```python
from build123d import *

# Parameters (mm, degrees)
SKETCH_4_W          = 88.9
SKETCH_4_H          = 88.9
SKETCH_4_R          = 1.5
SKETCH_4_W_2        = 38.1
SKETCH_4_H_2        = 3
SKETCH_4_W_3        = 3
SKETCH_4_H_3        = 38.1
EXTRUDE_1_DEPTH     = 3
SKETCH_6_W          = 88.9
SKETCH_6_H          = 3
EXTRUDE_2_DEPTH     = 24.13
SKETCH_7_W          = 3
SKETCH_7_H          = 7.62
CUT_EXTRUDE_1_DEPTH = 3


with BuildPart() as part:
    # 스케치4 → 보스-돌출1 (new body)
    with BuildSketch(Plane(origin=(0, 0, 0), x_dir=(1, 0, 0), z_dir=(0, 1, 0))):
        Rectangle(SKETCH_4_W, SKETCH_4_H)
        with Locations(Location((-41.275, 41.275, 0), (0, 0, 270))):
            Circle(SKETCH_4_R, mode=Mode.SUBTRACT)
        with Locations(Location((41.275, 41.275, 0), (0, 0, 270))):
            Circle(SKETCH_4_R, mode=Mode.SUBTRACT)
        with Locations(Location((41.275, -41.275, 0), (0, 0, 270))):
            Circle(SKETCH_4_R, mode=Mode.SUBTRACT)
        with Locations(Location((-41.275, -41.275, 0), (0, 0, 270))):
            Circle(SKETCH_4_R, mode=Mode.SUBTRACT)
        with Locations((0, 36.6)):
            Rectangle(SKETCH_4_W_2, SKETCH_4_H_2, mode=Mode.SUBTRACT)
        with Locations((36.6, 0)):
            Rectangle(SKETCH_4_W_3, SKETCH_4_H_3, mode=Mode.SUBTRACT)
        with Locations((0, -36.6)):
            Rectangle(SKETCH_4_W_2, SKETCH_4_H_2, mode=Mode.SUBTRACT)
        with Locations((-36.6, 0)):
            Rectangle(SKETCH_4_W_3, SKETCH_4_H_3, mode=Mode.SUBTRACT)
    extrude(amount=EXTRUDE_1_DEPTH)

    # 스케치6 → 보스-돌출2 (add)
    with BuildSketch(Plane(origin=(44.45, 0, 0), x_dir=(0, 0, -1), z_dir=(1, 0, 0))):
        with Locations((0, 1.5)):
            Rectangle(SKETCH_6_W, SKETCH_6_H)
    extrude(amount=EXTRUDE_2_DEPTH)

    # 스케치7 → 컷-돌출1 (cut)
    with BuildSketch(Plane(origin=(0, 3, 0), x_dir=(1, 0, 0), z_dir=(0, 1, 0))):
        with Locations((-13.1, -28.21025)):
            Rectangle(SKETCH_7_W, SKETCH_7_H)
    extrude(amount=-CUT_EXTRUDE_1_DEPTH, mode=Mode.SUBTRACT)


solid = part.part
```
Geometry check sheet. Reference: the model listing, model coordinates, mm. A direction names the side the tool comes from. Round coordinates to 2 decimals unless told otherwise and drop trailing zeros. Loops run counter-clockwise (first coordinate to the right, second up) from the corner with the lowest first, then second, coordinate; pieces in that order, holes last. Notation, with made-up numbers: (88.25, 49) - (143.25, 49) arc R23 ccw to (143.25, 75) - close; hole circle Ø6 at (11, -17). An arc over 180 degrees is marked (long way). Use a Markdown table: item, result.
Q1. Cross-section at C-C on y = 1.9. State how many separate pieces and enclosed holes the cut face has, plus the area to 3 significant figures.
Solutions:
| item | result |
|---|---|
| separate pieces | 1 |
| enclosed holes | 9 |
| area | 9,540 mm2 |
Q2. Cross-section at B-B on x = 8.5. Record the cut outline in (y, z).
Solutions:
| item | result |
|---|---|
| outline | (0, -44.45) - (3, -44.45) - (3, -38.1) - (0, -38.1) - close; (0, -35.1) - (3, -35.1) - (3, 35.1) - (0, 35.1) - close; (0, 38.1) - (3, 38.1) - (3, 44.45) - (0, 44.45) - close |
Q3. Material ranges on line 1 (Z direction, x = 4, y = 1.4); line 2 (X direction, y = 0.6, z = 19); line 3 (X direction, y = 2.4, z = -40.5), recorded low to high.
Solutions:
| item | result |
|---|---|
| line 1 | z = -44.45 to -38.1, -35.1 to 35.1, 38.1 to 44.45 |
| line 2 | x = -44.45 to -38.1, -35.1 to 35.1, 38.1 to 68.58 |
| line 3 | x = -44.45 to -42.56, -39.99 to 39.99, 42.56 to 68.58 |
Q4. Go/stop test with a flat-tipped pin: P1, Ø2.5, axis at x = -41.275, z = -41.275, coming from the +Y side. Record where the tip stops, or that it passes through.
Solutions:
| item | result |
|---|---|
| P1 | passes through |
Q5. Cross-section at A-A on z = 36.5. Record the cut outline in (x, y).
Solutions:
| item | result |
|---|---|
| outline | (-44.45, 0) - (-19.05, 0) - (-19.05, 3) - (-44.45, 3) - close; (19.05, 0) - (68.58, 0) - (68.58, 3) - (19.05, 3) - close |
Q6. Access from +Z, -Z, +X, -X, +Y, -Y to the whole of each face (thin tool, end or side, straight path). Record for faces 4 (the flat face through (19.05, 1, 37)), 5 (the flat face through (11, 1, 44.45)).
Solutions:
| item | result |
|---|---|
| face 4 | +Y, -Y |
| face 5 | +Z, +X, -X, +Y, -Y |
Q7. Draft check along Z on faces 1 (the flat face through (11, 0, 1)), 2 (the flat face through (-14.6, 2, 28)), 3 (the flat face through (11, 1, -44.45)). Enter one of: released by +Z, released by -Z, zero draft, split by the parting line, or undercut.
Solutions:
| item | result |
|---|---|
| face 1 | zero draft |
| face 2 | undercut |
| face 3 | released by -Z |
